The model under review builds one solid part; all positions refer to its coordinate system, in mm. Face numbers are marked on the shaded views. A direction names the side the tool comes from. Coordinates: 2 decimals unless noted, no trailing zeros. Order: outer loops, then holes, each group sorted by start corner. A loop starts at its lowest first (then second) coordinate and runs counter-clockwise, first axis right, second up. Notation, with made-up numbers: (54, 6.25) -> (94, 6.25) arc R20 cw to (94, 38.25) -> close; hole circle Ø6 at (69, 22.5). An arc over 180 degrees is marked (long way). Use one line per item in the form item = value. Start each with the question number.
(1) For the marked faces 1, 2, 3, 4 and 5, list the 3-axis set-ups (+Z, -Z, +X, -X, +Y, -Y) from which the entire face can be reached by the end or side of a thin tool; tool diameter is ignored.
(2) Take a section at D-D (y = -66). State the section outline as (x, z) points, then the cut area to 3 significant figures.
(3) Wall thickness on line 1 along X through (y, z) = (-27, -6.5); line 2 along Y through (x, z) = (-14, -6); line 3 along Z through (x, y) = (-28.5, -19.5): over which ranges is each line inside the solid? List them lowest first.
(4) Take a section at C-C (z = 11.5). State the section outline as (x, y) points.
(5) Take a section at A-A (y = -34). State the section outline as (x, z) points, then the cut area to 3 significant figures.
(6) Insertion check: pin 1 Ø4 at (y, z) = (-20.5, 2) entering from -X; pin 2 Ø14.5 at (x, z) = (-16, 1.5) entering from -Y; pin 3 Ø3.5 at (y, z) = (0, 5.5) entering from +X. Each pin has a flat end and moves straight along its axis. Give the tip position at first contact, or say it passes through.
(7) Take a section at B-B (x = -114). State the section outline as (y, z) points.
```python
from build123d import *

# Parameters (mm, degrees)
BOSS_EXTRUDE1_DEPTH = 15
BOSS_EXTRUDE2_DEPTH = 9
BOSS_EXTRUDE3_START = -3.5
SKETCH1_4_R         = 11
BOSS_EXTRUDE3_DEPTH = 5.5


with BuildPart() as part:
    # Sketch1 → Boss-Extrude1 (new, symmetric)
    with BuildSketch(Plane.XY):
        with BuildLine():
            ThreePointArc((-161.958144077, 21.543307087), (-152.82526794, -33.65504728), (-124.10035648, -81.666995927))
            ThreePointArc((-124.10035648, -81.666995927), (-91.629362444, -83.573444545), (-89.722913826, -51.102450509))
            ThreePointArc((-89.722913826, -51.102450509), (-109.638852439, -17.814166114), (-115.970979893, 20.456692913))
            ThreePointArc((-115.970979893, 20.456692913), (-138.421254898, 43.993582092), (-161.958144077, 21.543307087))
        make_face()
        with BuildLine():
            ThreePointArc((-122.969026617, 20.622047244), (-138.586609229, 36.995535368), (-154.960097353, 21.377952756))
            ThreePointArc((-154.960097353, 21.377952756), (-146.253422103, -31.244478407), (-118.869006511, -77.01586945))
            ThreePointArc((-118.869006511, -77.01586945), (-96.280488921, -78.342094576), (-94.954263795, -55.753576986))
            ThreePointArc((-94.954263795, -55.753576986), (-116.210698276, -20.224734987), (-122.969026617, 20.622047244))
        make_face(mode=Mode.SUBTRACT)
    extrude(amount=BOSS_EXTRUDE1_DEPTH, both=True)

    # Sketch1_3 → Boss-Extrude2 (add, symmetric)
    with BuildSketch(Plane.XY):
        with BuildLine():
            Line((-52, -44), (-23, -44))
            Line((-23, -44), (-23, 44))
            Line((-23, 44), (-138.964561985, 44))
            ThreePointArc((-138.964561985, 44), (-122.51013913, 37.070219927), (-115.970979893, 20.456692913))
            ThreePointArc((-115.970979893, 20.456692913), (-115.99647598, 18.856144662), (-115.997334395, 17.255393583))
            ThreePointArc((-115.997334395, 17.255393583), (-113.188190384, 24.141624797), (-106.322248233, 27))
            Line((-106.322248233, 27), (-65.39696962, 27))
            ThreePointArc((-65.39696962, 27), (-42.299981307, 11.567085809), (-47.71930009, -15.67766953))
            Line((-47.71930009, -15.67766953), (-78.190423053, -46.148792492))
            ThreePointArc((-78.190423053, -46.148792492), (-86.706172416, -49.345862018), (-94.717571561, -45.038110339))
            ThreePointArc((-94.717571561, -45.038110339), (-92.277527324, -48.11746068), (-89.722913826, -51.102450509))
            ThreePointArc((-89.722913826, -51.102450509), (-83.921522259, -67.059044464), (-90.648179186, -82.648179186))
            Line((-90.648179186, -82.648179186), (-52, -44))
        make_face()
    extrude(amount=BOSS_EXTRUDE2_DEPTH, both=True)

    # Sketch1_4 → Boss-Extrude3 (add, symmetric)
    with BuildSketch(Plane.XY.offset(BOSS_EXTRUDE3_START)):
        with BuildLine():
            Line((-23, -44), (0, -44))
            ThreePointArc((0, -44), (19.528931575, -39.428680317), (35, -26.664583252))
            Line((35, -26.664583252), (35, 26.664583252))
            ThreePointArc((35, 26.664583252), (19.528931575, 39.428680317), (0, 44))
            Line((0, 44), (-23, 44))
            Line((-23, 44), (-23, -44))
        make_face()
        Circle(SKETCH1_4_R, mode=Mode.SUBTRACT)
    extrude(amount=BOSS_EXTRUDE3_DEPTH, both=True)


solid = part.part
```
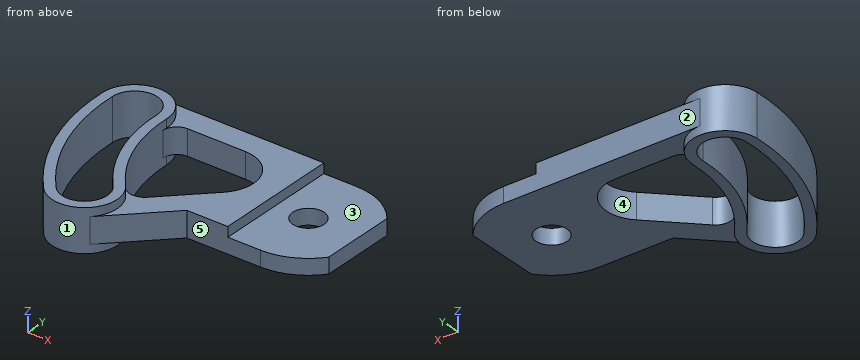
Findings:
q1.face_1 = none
q1.face_2 = +Z, -Z, +X, -X, +Y
q1.face_3 = +Z, +X, +Y, -Y
q1.face_4 = +Z, -Z
q1.face_5 = +Z, -Z, +X, -Y
q2.outline = (-136.27, -15) -> (-127.73, -15) -> (-127.73, 15) -> (-136.27, 15) -> close; (-90.92, -15) -> (-83.91, -15) -> (-83.91, -9) -> (-74, -9) -> (-74, 9) -> (-83.91, 9) -> (-83.91, 15) -> (-90.92, 15) -> close
q2.area = 645 mm²
q3.line_1 = -155.09 to -147.74, -113.47 to -105.76, -59.04 to 34.74
q3.line_2 = -44 to 44
q3.line_3 = -9 to 9
q4.outline = (-161.96, 21.54) arc R150 ccw to (-124.1, -81.67) arc R23 ccw to (-89.72, -51.1) arc R104 cw to (-115.97, 20.46) arc R23 ccw to start; hole (-154.96, 21.38) arc R143 ccw to (-118.87, -77.02) arc R16 ccw to (-94.95, -55.75) arc R111 cw to (-122.97, 20.62) arc R16 ccw to start
q5.outline = (-152.7, -15) -> (-145.21, -15) -> (-145.21, 15) -> (-152.7, 15) -> close; (-110.07, -15) -> (-102.07, -15) -> (-102.07, 15) -> (-110.07, 15) -> close; (-66.04, -9) -> (27.93, -9) -> (27.93, 2) -> (-23, 2) -> (-23, 9) -> (-66.04, 9) -> close
q5.area = 1,800 mm²
q6.pin_1 = -157.49
q6.pin_2 = -44
q6.pin_3 = -23
q7.outline = (-88.27, -15) -> (-80.73, -15) -> (-80.73, 15) -> (-88.27, 15) -> close; (-25.78, -15) -> (-2.3, -15) -> (-2.3, 15) -> (-25.78, 15) -> close; (23.21, -9) -> (44, -9) -> (44, 9) -> (23.21, 9) -> close
